For this review, take the finished solid that the model builds, in its own axes (mm). A direction names the side the tool comes from. Give positions to 0.01 mm unless a question says otherwise; leave off trailing zeros. Loops run counter-clockwise (first coordinate to the right, second up) from the corner with the lowest first, then second, coordinate; pieces in that order, holes last. Notation, with made-up numbers: (45.25, 59) - (63.25, 59) arc R27 ccw to (63.25, 75) - close; hole circle Ø10 at (74.25, -19). An arc over 180 degrees is marked (long way). Answer as CSV lines item,"result".
Solid Edge part; units mm, degrees
sketch "Sketch1" plane through (0, 0, 0) normal (0, 0, 1) x (1, 0, 0)
  circle A0 centre (0, 0) radius 8
  circle A1 centre (0, 0) radius 2.5
extrude "Protrusion1" add sketch "Sketch1" along normal blind 5
sketch "Sketch2" plane through (0, 0, 0) normal (1, 0, 0) x (0, 1, 0)
  line L0 (-6.6635, 5) -> (-6.6635, 4.0783)
  line L1 (-6.6635, 4.0783) -> (-3.8384, 4.0783)
  line L2 (-3.8384, 4.0783) -> (-3.8384, 5)
revolve "RevolvedCutout1" cut sketch "Sketch2" angle 360 about axis through (0, 0, -57) along (0, 0, 1) material side at (0, -6.6135, 4.5391)
mirror "Mirror1" about plane through (0, 0, 2.5) normal (0, 0, 1) of "RevolvedCutout1"
properties material "Stainless steel"
1) Machinability: for faces 1 (the flat face through (3, 0, 5)), 2 (the flat face through (-3, 3, 0.922)), 3 (the cylindrical face through (-3.747, 0.832, 4.546)), which of the approach directions +Z, -Z, +X, -X, +Y, -Y give a long, thin tool a straight path to every point of the face, cutting with its end or side? Answer none if there is none.
From the geometry:
face 1,"+Z, +X, -X, +Y, -Y"
face 2,"-Z"
face 3,"+Z"
2) Wall thickness on line 1 (Y direction, x = 0, z = 2.25); line 2 (Y direction, x = -0.75, z = 4.25); line 3 (Y direction, x = -5.5, z = 4.45): over which ranges is each line inside the solid? List them lowest first. Write a range as from..to.
From the geometry:
line 1,"y = -8..-2.5, 2.5..8"
line 2,"y = -7.96..-6.62, -3.76..-2.38, 2.38..3.76, 6.62..7.96"
line 3,"y = -5.81..-3.76, 3.76..5.81"
3) Consider section C-C on z = 0.3. Write out the cut boundary in (x, y).
From the geometry:
outline,"circle Ø16 at (0, 0); circle Ø7.68 at (0, 0); hole circle Ø13.33 at (0, 0); hole circle Ø5 at (0, 0)"
4) Consider section A-A on y = 0. Write out the cut boundary in (x, z).
From the geometry:
outline,"(-8, 0) - (-6.66, 0) - (-6.66, 0.92) - (-3.84, 0.92) - (-3.84, 0) - (-2.5, 0) - (-2.5, 5) - (-3.84, 5) - (-3.84, 4.08) - (-6.66, 4.08) - (-6.66, 5) - (-8, 5) - close; (2.5, 0) - (3.84, 0) - (3.84, 0.92) - (6.66, 0.92) - (6.66, 0) - (8, 0) - (8, 5) - (6.66, 5) - (6.66, 4.08) - (3.84, 4.08) - (3.84, 5) - (2.5, 5) - close"
5) Insertion check: P1, Ø1, axis at y = -4, z = 1.5, coming from the +X side; P2, Ø3, axis at y = -6, z = 2, coming from the -X side; P3, Ø3, axis at x = -6, z = 2.5, coming from the +Y side. Each pin has a flat end and moves straight along its axis. Give the tip position at first contact, or say it passes through.
From the geometry:
P1,"stops at x = 7.19"
P2,"stops at x = -6.61"
P3,"stops at y = 6.61"
6) Draft analysis for pull direction X (two halves, no side actions). For faces 4 (the cylindrical face through (3.747, 0.832, 0.454)), 5 (the cylindrical face through (-1.73, 7.81, 2.46)), 6 (the cylindrical face through (-4.504, 4.911, 4.533)), 7 (the flat face through (-2, 7, 0)), state which applies: pulls with the +X half, pulls with the -X half, needs draft (parallel to the pull), parting line crosses it, or undercut.
From the geometry:
face 4,"undercut"
face 5,"parting line crosses it"
face 6,"undercut"
face 7,"needs draft"
7) Consider section D-D on z = 1.95. Write out the cut boundary in (x, y).
From the geometry:
outline,"circle Ø16 at (0, 0); hole circle Ø5 at (0, 0)"
